For this review, take the finished solid that the model builds, in its own axes (mm). A direction names the side the tool comes from. Round coordinates to 2 decimals unless told otherwise and drop trailing zeros. Write each loop counter-clockwise with the first axis right and the second up, starting at its lowest first coordinate (ties: lowest second). Pieces come first, ordered by that corner, then holes. Notation, with made-up numbers: M 66,55 L 109,55 A35 ccw 109,94 Z; hole C -27,83 d1. An arc over 180 degrees is marked long. Answer in a Markdown table with one row per item.
Autodesk Inventor part; units mm, degrees
ref_plane "YZ Plane" through (0, 0, 0) normal (1, 0, 0) x (0, 1, 0)
ref_plane "XZ Plane" through (0, 0, 0) normal (0, 1, 0) x (-1, 0, 0)
ref_plane "XY Plane" through (0, 0, 0) normal (0, 0, 1) x (1, 0, 0)
sketch "Szkic1" plane through (0, 0, 0) normal (0, 0, 1) x (1, 0, 0)
  line L0 (-15.1556, -3.6171) -> (-15.1556, -6.6171)
  line L1 (-15.1556, -6.6171) -> (10.8444, -6.6171)
  line L2 (10.8444, -6.6171) -> (10.8444, 23.3829)
  line L3 (7.8444, 20.3829) -> (7.8444, -3.6171)
  line L4 (7.8444, -3.6171) -> (-15.1556, -3.6171)
  line L5 (-15.1556, 23.3829) -> (-15.1556, 20.3829)
  line L6 (-15.1556, 20.3829) -> (7.8444, 20.3829)
  line L7 (-15.1556, 23.3829) -> (10.8444, 23.3829)
  point P0 (0, 0)
  dimension "d1" = 26
  dimension "d2" = 30
  dimension "d87" = 3
  dimension "d88" = 24
  dimension "d89" = 3
  dimension "d90" = 3
extrude "Wyciągnięcie proste1" add sketch "Szkic1" along normal blind 36
fillet "Zaokrąglenie1" radius 1 2 edges at (7.8444, -3.6171, 18) (7.8444, 20.3829, 18)
chamfer "Faza4" distance 1.5 angle 45 4 edges at (-15.1556, -5.1171, 36) (-15.1556, -5.1171, 0) (-15.1556, 21.8829, 36) (-15.1556, 21.8829, 0)
fillet "Zaokrąglenie5" radius 2 2 edges at (10.8444, 8.3829, 36) (10.8444, 8.3829, 0)
sketch "Szkic7" plane through (-15.1556, -6.6171, 1.5) normal (0, -1, 0) x (1, 0, 0)
  arc A0 (24, -1.5) -> (26, 0.5) centre (24, 0.5) ccw
  line L0 (26, 0.5) -> (26, 32.5)
  arc A1 (26, 32.5) -> (24, 34.5) centre (24, 32.5) ccw
  line L1 (1.5, 34.5) -> (24, 34.5)
  line L2 (0, 33) -> (1.5, 34.5)
  line L3 (0, 0) -> (0, 33)
  line L4 (1.5, -1.5) -> (0, 0)
  line L5 (1.5, -1.5) -> (24, -1.5)
  line L6 (23, 34.5) -> (23, -1.5)
  point P0 (15.1556, -1.5)
  point P1 (19, 6.25)
  point P2 (4, 6.25)
  point P3 (4, 26.75)
  point P4 (19, 26.75)
  dimension "d95" = 4
  dimension "d96" = 4
  dimension "d97" = 4
  dimension "d98" = 4
  dimension "d99" = 7.75
  dimension "d100" = 7.75
  dimension "d101" = 7.75
  dimension "d102" = 7.75
hole "Otwór5" at (3.8444, -6.6171, 7.75) at (-11.1556, -6.6171, 7.75) at (-11.1556, -6.6171, 28.25) at (3.8444, -6.6171, 28.25) direction (0, 1, 0) diameter 3 depth 8 tip angle 118
sketch "Szkic8" plane through (-15.1556, 23.3829, 34.5) normal (0, 1, 0) x (1, 0, 0)
  arc A0 (26, 32.5) -> (24, 34.5) centre (24, 32.5) ccw
  line L0 (24, 34.5) -> (1.5, 34.5)
  line L1 (0, 33) -> (1.5, 34.5)
  line L2 (0, 33) -> (0, 0)
  line L3 (1.5, -1.5) -> (0, 0)
  line L4 (24, -1.5) -> (1.5, -1.5)
  arc A1 (24, -1.5) -> (26, 0.5) centre (24, 0.5) ccw
  line L5 (26, 32.5) -> (26, 0.5)
  line L6 (23, 34.5) -> (23, -1.5)
  point P0 (15.1556, 34.5)
  point P1 (11.5, 26.5)
  point P2 (11.5, 6.5)
  dimension "d110" = 11.5
  dimension "d111" = 23
  dimension "d112" = 11.5
  dimension "d113" = 20
  dimension "d114" = 36
  dimension "d115" = 8
hole "Otwór6" at (-3.6556, 23.3829, 8) at (-3.6556, 23.3829, 28) direction (0, -1, 0) diameter 4 depth 8 tip angle 118
sketch "Szkic9" plane through (-15.1556, -6.6171, 1.5) normal (0, -1, 0) x (1, 0, 0)
  circle A0 centre (11.5, 6.5) radius 2
  circle A1 centre (11.5, 26.5) radius 2
  circle A2 centre (11.5, 6.5) radius 1.5
  circle A3 centre (11.5, 26.5) radius 1.5
  point P0 (15.1556, -1.5)
  dimension "d123" = 3
  dimension "d124" = 3
extrude "Wyciągnięcie proste4" cut sketch "Szkic9" against normal blind 10 contours A2 | A3
equation "\"d88\" = d2 - 2 * d87"
properties part number "CNCM_ALU_Y_Axis_Belt_Mount_Bracket"
Q1. Insertion check: P1, Ø3, axis at y = 11.5, z = 20, coming from the -X side; P2, Ø2.5, axis at x = -11.16, z = 7.75, coming from the -Y side. Each pin has a flat end and moves straight along its axis. Give the tip position at first contact, or say it passes through.
Found:
| item | result |
|---|---|
| P1 | x = 7.84 |
| P2 | y = 20.38 |
Q2. Take a section at C-C (x = -11.75). State the section outline as (y, z) points, then the cut area to 3 significant figures.
Found:
| item | result |
|---|---|
| outline | M -6.62,0 L -3.62,0 L -3.62,6.37 L -6.62,6.37 Z; M -6.62,9.13 L -3.62,9.13 L -3.62,26.87 L -6.62,26.87 Z; M -6.62,29.63 L -3.62,29.63 L -3.62,36 L -6.62,36 Z; M 20.38,0 L 23.38,0 L 23.38,36 L 20.38,36 Z |
| area | 199 mm² |
Q3. Take a section at A-A (x = -6.5). State the section outline as (y, z) points, then the cut area to 3 significant figures.
Found:
| item | result |
|---|---|
| outline | M -6.62,0 L -3.62,0 L -3.62,36 L -6.62,36 Z; M 20.38,0 L 23.38,0 L 23.38,36 L 20.38,36 Z |
| area | 216 mm² |
Q4. Machinability: for faces 5 (the face through (-4, -3.617, 18)), 6 (the face through (-4.256, 21.862, 29.908)), 7 (the face through (-10.24, -5.1, 8.94)), 8 (the face through (10.844, 8, 18)), 9 (the face through (-14.416, -5.096, 0.761)), which of the approach directions +Z, -Z, +X, -X, +Y, -Y give a long, thin tool a straight path to every point of the face, cutting with its end or side? Answer none if there is none.
Found:
| item | result |
|---|---|
| face 5 | +Z, -Z, -X |
| face 6 | +Y |
| face 7 | -Y |
| face 8 | +Z, -Z, +X, +Y, -Y |
| face 9 | -Z, -X, +Y, -Y |
Q5. Mouldability with a two-part tool opening along Z and no side actions: class faces 1 (the face through (3.78, -5.1, 29.75)), 2 (the face through (-15.156, -5, 18)), 3 (the face through (-14.416, 21.904, 0.761)), 4 (the face through (-14.395, -5.138, 35.26)) as +Z half, -Z half, draft (parallel to the pull), parting line (faces both ways), or undercut.
Found:
| item | result |
|---|---|
| face 1 | undercut |
| face 2 | draft |
| face 3 | -Z half |
| face 4 | +Z half |
Q6. Take a section at B-B (z = 8.5). State the section outline as (x, y) points, then the cut area to 3 significant figures.
Found:
| item | result |
|---|---|
| outline | M -15.16,-6.62 L -12.45,-6.62 L -12.45,-3.62 L -15.16,-3.62 Z; M -15.16,20.38 L -5.59,20.38 L -5.59,23.38 L -15.16,23.38 Z; M -9.86,-6.62 L -5.07,-6.62 L -5.07,-3.62 L -9.86,-3.62 Z; M -2.24,-6.62 L 2.55,-6.62 L 2.55,-3.62 L -2.24,-3.62 Z; M -1.72,20.38 L 6.84,20.38 A1 cw 7.84,19.38 L 7.84,-2.62 A1 cw 6.84,-3.62 L 5.14,-3.62 L 5.14,-6.62 L 10.84,-6.62 L 10.84,23.38 L -1.72,23.38 Z |
| area | 193 mm² |
Q7. Take a section at D-D (z = 16). State the section outline as (x, y) points, then the cut area to 3 significant figures.
Found:
| item | result |
|---|---|
| outline | M -15.16,-6.62 L 10.84,-6.62 L 10.84,23.38 L -15.16,23.38 L -15.16,20.38 L 6.84,20.38 A1 cw 7.84,19.38 L 7.84,-2.62 A1 cw 6.84,-3.62 L -15.16,-3.62 Z |
| area | 228 mm² |
Q8. For probe 1 along Y at (x, z) = (6.75, 22); probe 2 along X at (y, z) = (-4.45, 7.75); probe 3 along X at (y, z) = (9.5, 15.5), list the stretches that pass through material, from the lowest coordinate up.
Found:
| item | result |
|---|---|
| probe 1 | -6.62 to -3.62, 20.38 to 23.38 |
| probe 2 | -15.16 to -12.66, -9.66 to -5.13, -2.18 to 2.34, 5.34 to 10.84 |
| probe 3 | 7.84 to 10.84 |
